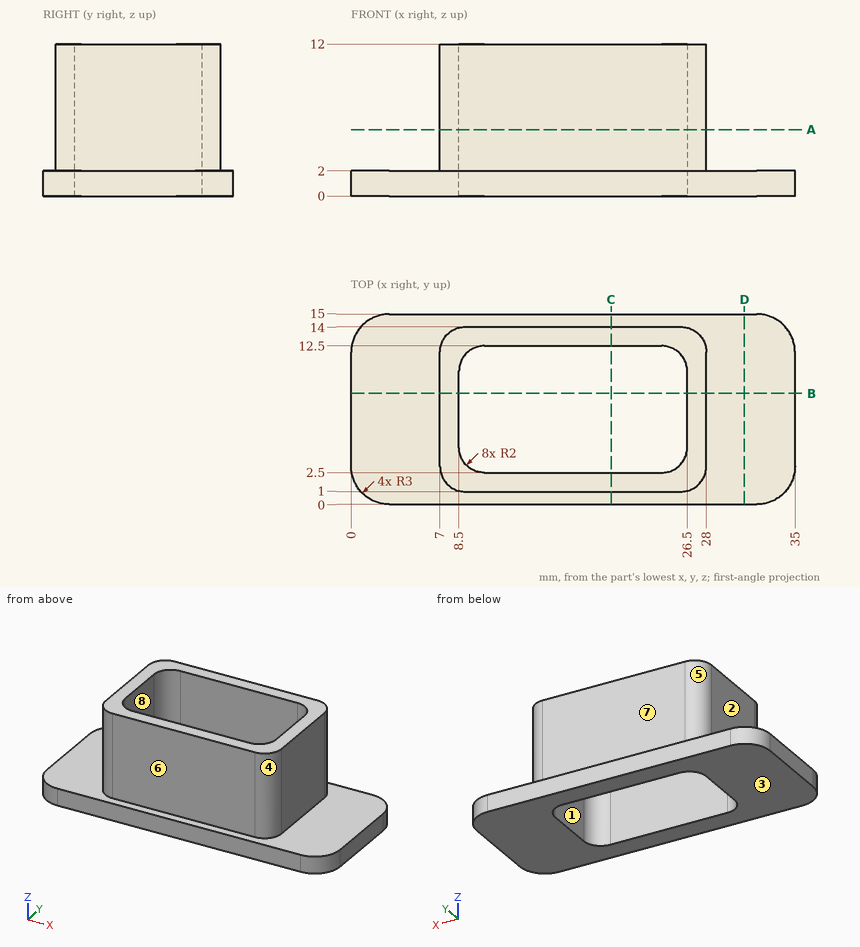
Could you check a few things on this drawing? It's one solid part, dimensions in mm from its lowest x, y, z. A direction names the side the tool comes from. Round coordinates to 2 decimals unless told otherwise and drop trailing zeros. Loops run counter-clockwise (first coordinate to the right, second up) from the corner with the lowest first, then second, coordinate; pieces in that order, holes last. Notation, with made-up numbers: M -2.75,48.25 L 11.25,48.25 A13 ccw 11.25,65.25 Z; hole C 4,30.25 d7. An arc over 180 degrees is marked long. Write each question's results on one line, items separated by ' | '. Start each with the question number.
(1) I want a section at D-D (x = 31). Please give me the cut outline in (y, z).
(2) I want a section at C-C (x = 20.5). Please give me the cut outline in (y, z).
(3) Will these pins go through, and if not, where does the flat tip stop? P1, Ø2.5, axis at y = 6.5, z = 9, coming from the +X side; P2, Ø6.5, axis at y = 7.5, z = 6, coming from the -X side.
(4) Thinking about a two-plate mould opening in X: for the marked faces 1, 2 and 3, which applies, pulls with the +X half, pulls with the -X half, needs draft (parallel to the pull), parting line crosses it, or undercut?
(5) On a 3-axis mill with a long thin cutter (end or side, diameter ignored), from which of +Z, -Z, +X, -X, +Y, -Y can I reach the whole of each face in a straight line? I mean the marked faces 4, 5, 6, 7 and 8. Say none if no direction works.
(6) If I drill on probe 1 along X at (y, z) = (6.25, 4.5); probe 2 along X at (y, z) = (4.5, 1.25); probe 3 along Y at (x, z) = (18, 9.5), over which ranges is the centre line in solid material (lowest first)? Write a range as from..to.
(7) I want a section at B-B (y = 8.75). Please give me the cut outline in (x, z).
(8) I want a section at A-A (z = 5.25). Please give me the cut outline in (x, y), then the cut area to 3 significant figures.
Solved:
1) outline: M 0,0 L 15,0 L 15,2 L 0,2 Z
2) outline: M 0,0 L 2.5,0 L 2.5,12 L 1,12 L 1,2 L 0,2 Z; M 12.5,0 L 15,0 L 15,2 L 14,2 L 14,12 L 12.5,12 Z
3) P1: stops at x = 28 | P2: stops at x = 7
4) face 1: undercut | face 2: pulls with the -X half | face 3: needs draft
5) face 4: +Z, +X, -Y | face 5: +Z, -X, +Y | face 6: +Z, +X, -X, -Y | face 7: +Z, +X, -X, +Y | face 8: +Z, -Z
6) probe 1: x = 7..8.5, 26.5..28 | probe 2: x = 0..8.5, 26.5..35 | probe 3: y = 1..2.5, 12.5..14
7) outline: M 0,0 L 8.5,0 L 8.5,12 L 7,12 L 7,2 L 0,2 Z; M 26.5,0 L 35,0 L 35,2 L 28,2 L 28,12 L 26.5,12 Z
8) outline: M 7,3 A2 ccw 9,1 L 26,1 A2 ccw 28,3 L 28,12 A2 ccw 26,14 L 9,14 A2 ccw 7,12 Z; hole M 8.5,4.5 A2 ccw 10.5,2.5 L 24.5,2.5 A2 ccw 26.5,4.5 L 26.5,10.5 A2 ccw 24.5,12.5 L 10.5,12.5 A2 ccw 8.5,10.5 Z | area: 93.0 mm²
